from build123d import *

# Parameters (mm, degrees)
SKETCH1_R           = 1.355900406
BOSS_EXTRUDE1_DEPTH = 1.5875
SKETCH2_R           = 3.175
BOSS_EXTRUDE2_DEPTH = 1.5875
SKETCH3_R           = 1.524
CUT_EXTRUDE1_DEPTH  = 436.184338179
CUT_EXTRUDE2_DEPTH  = 436.184338179
SKETCH5_W           = 2.0955
SKETCH5_H           = 13.208
BOSS_EXTRUDE3_DEPTH = 1.5875


with BuildPart() as part:
    # Sketch1 → Boss-Extrude1 (new body)
    with BuildSketch(Plane.XY):
        with BuildLine():
            Line((-301.9473, 111.74645), (-305.87795, 115.6771))
            Line((-305.87795, 115.6771), (-316.1078, 115.6771))
            Line((-316.1078, 115.6771), (-316.1078, 128.8851))
            Line((-316.1078, 128.8851), (-305.87795, 128.8851))
            Line((-305.87795, 128.8851), (-301.9473, 132.81575))
            Line((-301.9473, 132.81575), (-301.9473, 150.9704))
            ThreePointArc((-301.9473, 150.9704), (-303.063223164, 153.664476836), (-305.7573, 154.7804))
            Line((-305.7573, 154.7804), (-397.247125, 154.7804))
            ThreePointArc((-397.247125, 154.7804), (-399.946077222, 153.659592612), (-401.0571, 150.956597849))
            Line((-401.0571, 150.956597849), (-401.0571, 148.341))
            Line((-401.0571, 148.341), (-399.1521, 148.341))
            Line((-399.1521, 148.341), (-399.1521, 95.6449))
            Line((-399.1521, 95.6449), (-401.0571, 95.6449))
            Line((-401.0571, 95.6449), (-401.0571, 91.659304166))
            ThreePointArc((-401.0571, 91.659304166), (-399.951018769, 88.947400452), (-397.2472, 87.8217))
            Line((-397.2472, 87.8217), (-378.5565, 87.8217))
            Line((-378.5565, 87.8217), (-368.3165, 91.1883))
            Line((-368.3165, 91.1883), (-315.9973, 91.1883))
            Line((-315.9973, 91.1883), (-305.7573, 87.8217))
            ThreePointArc((-305.7573, 87.8217), (-303.063223164, 88.937623164), (-301.9473, 91.6317))
            Line((-301.9473, 91.6317), (-301.9473, 111.74645))
        make_face()
        with Locations((-305.7573, 91.6317)):
            Circle(SKETCH1_R, mode=Mode.SUBTRACT)
        with Locations((-305.7573, 150.9704)):
            Circle(SKETCH1_R, mode=Mode.SUBTRACT)
        with Locations((-397.247125, 150.9704)):
            Circle(SKETCH1_R, mode=Mode.SUBTRACT)
        with Locations((-397.2472, 91.6317)):
            Circle(SKETCH1_R, mode=Mode.SUBTRACT)
    extrude(amount=BOSS_EXTRUDE1_DEPTH)

    # Sketch2 → Boss-Extrude2 (add)
    # profile 1 of 2: a face of its own
    with BuildSketch(Plane.XY.offset(1.5875)):
        with BuildLine():
            Line((-361.0272, 159.40105), (-361.0272, 154.7804))
            Line((-361.0272, 154.7804), (-341.9772, 154.7804))
            Line((-341.9772, 154.7804), (-341.9772, 159.40105))
            ThreePointArc((-341.9772, 159.40105), (-351.5022, 168.92605), (-361.0272, 159.40105))
        make_face()
        with Locations((-351.5022, 159.40105)):
            Circle(SKETCH2_R, mode=Mode.SUBTRACT)
    # profile 2 of 2: a face of its own
    with BuildSketch(Plane.XY.offset(1.5875)):
        with BuildLine():
            Line((-341.9772, 91.1883), (-361.0272, 91.1883))
            Line((-361.0272, 91.1883), (-361.0272, 83.20105))
            ThreePointArc((-361.0272, 83.20105), (-351.5022, 73.67605), (-341.9772, 83.20105))
            Line((-341.9772, 83.20105), (-341.9772, 91.1883))
        make_face()
        with Locations((-351.5022, 83.20105)):
            Circle(SKETCH2_R, mode=Mode.SUBTRACT)
    extrude(amount=-BOSS_EXTRUDE2_DEPTH)

    # Sketch3 → Cut-Extrude1 (cut, through all)
    with BuildSketch(Plane.XY.offset(1.5875)):
        with Locations((-397.247125, 150.9704)):
            Circle(SKETCH3_R)
        with Locations((-305.7573, 150.9704)):
            Circle(SKETCH3_R)
        with Locations((-305.7573, 91.6317)):
            Circle(SKETCH3_R)
        with Locations((-397.2472, 91.6317)):
            Circle(SKETCH3_R)
    extrude(amount=-CUT_EXTRUDE1_DEPTH, mode=Mode.SUBTRACT)

    # Sketch4 → Cut-Extrude2 (cut, through all)
    with BuildSketch(Plane.XY.offset(1.5875)):
        Polygon((-301.9473, 136.11775), (-305.87795, 132.1871), (-314.0123, 132.1871), (-314.0123, 111.1051), (-305.87795, 111.1051), (-301.9473, 107.17445), align=None)
    extrude(amount=-CUT_EXTRUDE2_DEPTH, mode=Mode.SUBTRACT)

    # Sketch5 → Boss-Extrude3 (add)
    with BuildSketch(Plane.XY.offset(1.5875)):
        with Locations((-315.06005, 122.2811)):
            Rectangle(SKETCH5_W, SKETCH5_H)
    extrude(amount=-BOSS_EXTRUDE3_DEPTH)


solid = part.part
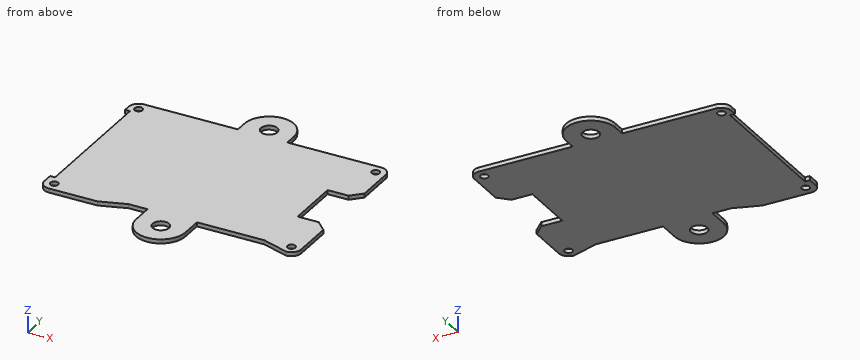
Model file for the job. Use its own axes, mm. Give positions to 0.01 mm unless a question says otherwise; leave off trailing zeros. Loops run counter-clockwise (first coordinate to the right, second up) from the corner with the lowest first, then second, coordinate; pieces in that order, holes last.
1) Saw through at C-C (y = 127.5). Write the cut outline in (x, z).
2) Wall check: line 1 (Y direction, x = -351.5, z = 0.35); line 2 (X direction, y = 151.5, z = 0.35); line 3 (Y direction, x = -386.5, z = 1.25). Give the ranges that are in metal, low to high.
3) Saw through at A-A (x = -308.5). Write the cut outline in (y, z), plus the area to 3 significant figures.
4) Flat gauge pins, fed straight in: pin 1 Ø0.8 at (y, z) = (123.5, 1) entering from -X; pin 2 Ø0.8 at (y, z) = (156.5, 0.5) entering from -X; pin 3 Ø4 at (x, y) = (-351.5, 159.4) entering from +Z; pin 4 Ø0.8 at (y, z) = (120, 0.5) entering from +X. Where does each tip first touch, or does it go through?
5) Saw through at B-B (y = 89). Write the cut outline in (x, z).
6) Saw through at D-D (z = 1). Count the separate pieces of the cut face and the enclosed holes in it, plus the area to 3 significant figures.
Answer block:
1. outline: (-399.15, 0) - (-314.01, 0) - (-314.01, 1.59) - (-399.15, 1.59) - close
2. line 1: y = 73.68 to 80.03, 86.38 to 156.23, 162.58 to 168.93
2. line 2: x = -401.02 to -398.68, -395.82 to -307.19, -304.33 to -301.98
2. line 3: y = 87.82 to 154.78
3. outline: (88.72, 0) - (111.11, 0) - (111.11, 1.59) - (88.72, 1.59) - close; (132.19, 0) - (154.78, 0) - (154.78, 1.59) - (132.19, 1.59) - close
3. area: 71.4 mm2
4. pin 1: stops at x = -399.15
4. pin 2: stops at x = -361.03
4. pin 3: passes through
4. pin 4: stops at x = -314.01
5. outline: (-400, 0) - (-374.97, 0) - (-374.97, 1.59) - (-400, 1.59) - close; (-361.03, 0) - (-341.98, 0) - (-341.98, 1.59) - (-361.03, 1.59) - close; (-309.34, 0) - (-303, 0) - (-303, 1.59) - (-309.34, 1.59) - close
6. separate pieces: 1
6. enclosed holes: 6
6. area: 6,480 mm2
